Can you work these out from the model? Positions are in its coordinate system, mm. A direction names the side the tool comes from. Give positions to 0.01 mm unless a question says otherwise; leave off trailing zeros. Loops run counter-clockwise (first coordinate to the right, second up) from the corner with the lowest first, then second, coordinate; pieces in that order, holes last. Notation, with made-up numbers: (28, 46) - (66, 46) arc R11 cw to (66, 62) - close; hole circle Ø7 at (24.25, 60.5). An arc over 180 degrees is marked (long way). Answer as a JSON object with one key per item and string values.
```python
from build123d import *

# Parameters (mm, degrees)
SKETCH_14_W     = 40
SKETCH_14_H     = 3
EXTRUDE_4_DEPTH = 30
FILLET_1_R      = 10
FILLET_3_R      = 1
SKETCH_15_W     = 3
SKETCH_15_H     = 34.674561042
EXTRUDE_1_DEPTH = 20


with BuildPart() as part:
    # 草图14 → 拉伸-薄壁4 (new body)
    with BuildSketch(Plane.XY):
        with Locations((0, -10.200267181)):
            Rectangle(SKETCH_14_W, SKETCH_14_H)
    extrude(amount=EXTRUDE_4_DEPTH)

    # 圆角1
    fillet_1_edges = [part.edges().sort_by_distance(p)[0] for p in [
        (-20, -10.200267181, 30),
    ]]
    fillet(fillet_1_edges, radius=FILLET_1_R)

    # 圆角3
    fillet_3_edges = [part.edges().sort_by_distance(p)[0] for p in [
        (0, -11.700267181, 0),
    ]]
    fillet(fillet_3_edges, radius=FILLET_3_R)

    # 草图15 → 凸台-拉伸1 (add, symmetric)
    with BuildSketch(Plane(origin=(0, 0, 0), x_dir=(0, 0, -1), z_dir=(1, 0, 0))):
        with Locations((-1.5, 8.63701334)):
            Rectangle(SKETCH_15_W, SKETCH_15_H)
    extrude(amount=EXTRUDE_1_DEPTH, both=True)


solid = part.part
```
1) I need wall thicknesses on L1, parallel to Y at x = -17, z = 24.75; L2, parallel to Z at x = 9.5, y = -4.5; L3, parallel to X at y = -10, z = 26.75. Which ranges of each line are inside material? Lowest first, please.
Check sheet entries:
{"L1": "-11.7 to -8.7", "L2": "0 to 3", "L3": "-17.38 to 20"}
2) Which directions (+Z, -Z, +X, -X, +Y, -Y) give clear straight access to the entire face, cutting with the end or side of a thin tool? Please do faces 1 (the flat face through (0, -8.7, 16)), 2 (the flat face through (-20, 1.6, 2.6)).
Check sheet entries:
{"face 1": "+Z, +X, -X, +Y", "face 2": "+Z, -Z, -X, +Y, -Y"}
3) Imagine slicing it at B-B on z = 12.5. Write out the boundary of the cut face in (x, y).
Check sheet entries:
{"outline": "(-20, -11.7) - (20, -11.7) - (20, -8.7) - (-20, -8.7) - close"}
4) Imagine slicing it at C-C on y = 19. Write out the boundary of the cut face in (x, z), and give its area (3 significant figures).
Check sheet entries:
{"outline": "(-20, 0) - (20, 0) - (20, 3) - (-20, 3) - close", "area": "120 mm2"}
5) Imagine slicing it at A-A on x = 8.5. Write out the boundary of the cut face in (y, z), and give its area (3 significant figures).
Check sheet entries:
{"outline": "(-11.7, 1) arc R1 ccw to (-10.7, 0) - (25.97, 0) - (25.97, 3) - (-8.7, 3) - (-8.7, 30) - (-11.7, 30) - close", "area": "194 mm2"}
6) I'm going to push flat-ended pins straight in: P1, Ø12, axis at x = -13, y = 5, coming from the +Z side; P2, Ø3, axis at x = 14, z = 16.5, coming from the +Y side. Where does each tip first touch, or does it pass through?
Check sheet entries:
{"P1": "z = 3", "P2": "y = -8.7"}
7) Imagine slicing it at D-D on x = -11. Write out the boundary of the cut face in (y, z), and give its area (3 significant figures).
Check sheet entries:
{"outline": "(-11.7, 1) arc R1 ccw to (-10.7, 0) - (25.97, 0) - (25.97, 3) - (-8.7, 3) - (-8.7, 29.95) - (-11.7, 29.95) - close", "area": "194 mm2"}
